Geometry: final body of the model. Coordinates: model frame, mm. A direction names the side the tool comes from. Round coordinates to 2 decimals unless told otherwise and drop trailing zeros. Write each loop counter-clockwise with the first axis right and the second up, starting at its lowest first coordinate (ties: lowest second). Pieces come first, ordered by that corner, then holes. Notation, with made-up numbers: (60, 72) - (119, 72) arc R12 ccw to (119, 76) - close; hole circle Ø9 at (-27.75, -9.75). An arc over 180 degrees is marked (long way). Write each question's results on one line, items separated by ' | '.
from build123d import *

# Parameters (mm, degrees)
F1_DEPTH = 63.5
F0_W     = 24.663166
F0_H     = 19.05
F2_DEPTH = 25.4
F3_DEPTH = 7.9375
F4_R     = 6.35


with BuildPart() as f1:
    # F0 (on Front) → F1 (new body, symmetric)
    with BuildSketch(Plane.XZ):
        Polygon((-41.275, 9.525), (-41.275, -9.525), (41.275, -9.525), (41.275, 9.525), (22.225, 9.525), align=None)
    extrude(amount=F1_DEPTH, both=True)

    # F0 (on Front) → F2 (join, symmetric)
    with BuildSketch(Plane.XZ):
        with BuildLine():
            Line((22.225, 9.525), (41.275, 9.525))
            Line((41.275, 9.525), (41.275, 27.0002))
            ThreePointArc((41.275, 27.0002), (45.92468, 38.22552), (57.15, 42.8752))
            Line((57.15, 42.8752), (60.325, 42.8752))
            Line((60.325, 42.8752), (60.325, 61.9252))
            Line((60.325, 61.9252), (57.15, 61.9252))
            ThreePointArc((57.15, 61.9252), (32.454296, 51.695904), (22.225, 27.0002))
            Line((22.225, 27.0002), (22.225, 9.525))
        make_face()
        with Locations((72.656583, 52.4002)):
            Rectangle(F0_W, F0_H)
    extrude(amount=F2_DEPTH, both=True)

    # F0 (on Front) → F3 (join, symmetric)
    with BuildSketch(Plane.XZ):
        with BuildLine():
            add(Edge.make_bspline(
                [(-41.275, 9.525), (-41.275, 30.556278), (7.645971, 61.9252), (57.15, 61.9252)],
                knots=[0, 0, 0, 0, 111.504536, 111.504536, 111.504536, 111.504536], degree=3))
            Line((-41.275, 9.525), (22.225, 9.525))
            Line((22.225, 9.525), (22.225, 27.0002))
            ThreePointArc((22.225, 27.0002), (32.454296, 51.695904), (57.15, 61.9252))
        make_face()
    extrude(amount=F3_DEPTH, both=True)

    # F4
    f4_edges = [f1.edges().sort_by_distance(p)[0] for p in [
        (-41.275, -63.5, 0),
        (41.275, -63.5, 0),
    ]]
    fillet(f4_edges, radius=F4_R)


solid = f1.part
Q1. Section query C-C, the plane x = 72. Return loops of the section in (y, z).
Answer block:
outline: (-25.4, 42.88) - (25.4, 42.88) - (25.4, 61.93) - (-25.4, 61.93) - close
Q2. Access query for faces 1 (the flat face through (46, 25.4, 42)), 2 (the cylindrical face through (32.73, -16.79, 51.97)), 3 (the flat face through (22.225, 17, 18)), 4 (the flat face through (46, -25.4, 42)). Directions: +Z, -Z, +X, -X, +Y, -Y. A direction counts if a zero-diameter tool reaches every point of the face in a straight line with its end or side. Return the directions, or none.
Answer block:
face 1: +Z, +X, -X, +Y | face 2: +Z, -X, -Y | face 3: +Z, -X, +Y | face 4: +Z, +X, -X, -Y
Q3. Section query B-B, the plane y = 27. Return loops of the section in (x, z) (3 decimals).
Answer block:
outline: (-41.275, -9.525) - (41.275, -9.525) - (41.275, 9.525) - (-41.275, 9.525) - close
Q4. Section query A-A, the plane z = 3. Return loops of the section in (x, y) (3 decimals), plus the area to 3 significant figures.
Answer block:
outline: (-41.275, -57.15) arc R6.35 ccw to (-34.925, -63.5) - (34.925, -63.5) arc R6.35 ccw to (41.275, -57.15) - (41.275, 63.5) - (-41.275, 63.5) - close | area: 10,500 mm2
Q5. Mould query, pull axis X, two halves, no side actions, for faces 5 (the flat face through (1, 35, 9.525)), 6 (the cylindrical face through (39.365, -61.689, 0.133)), 7 (the cylindrical face through (32.73, 16.55, 51.97)). Classes: pulls with the +X half, pulls with the -X half, needs draft (parallel to the pull), parting line crosses it, or undercut.
Answer block:
face 5: needs draft | face 6: pulls with the +X half | face 7: pulls with the -X half
Q6. Ray query, line 1 along Z through (x, y) = (-3, 48) (3 decimals); line 2 along X through (y, z) = (-15, 11.5) (3 decimals); line 3 along X through (y, z) = (-36, 7) (3 decimals). Return the intervals inside material, ascending.
Answer block:
line 1: -9.525 to 9.525 | line 2: 22.225 to 41.275 | line 3: -41.275 to 41.275
Q7. Pin query (flat end, axial travel): pin 1 (8 mm diameter, centred on x = 11, z = 18, fed in from -Y); pin 2 (6 mm diameter, centred on x = -13, z = 11.5, fed in from +Y); pin 3 (15.5 mm diameter, centred on x = 58.5, z = 41.5, fed in from -Y); pin 4 (12 mm diameter, centred on y = -25.5, z = 23, fed in from +X). Return the tip coordinate at first contact, or that it passes through.
Answer block:
pin 1: y = -7.94 | pin 2: y = 63.5 | pin 3: y = -25.4 | pin 4: x = 41.4
